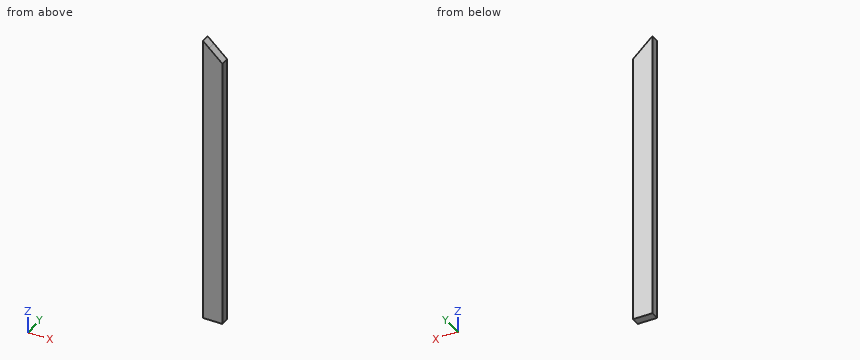
```python
from build123d import *

# Parameters (mm, degrees)
F0_W     = 88.9
F0_H     = 38.1
F1_DEPTH = 1371.6
F3_DEPTH = 38.101


with BuildPart() as f1:
    # F0 (on Top) → F1 (new body)
    with BuildSketch(Plane.XY):
        with Locations((44.45, 19.05)):
            Rectangle(F0_W, F0_H)
    extrude(amount=F1_DEPTH)

    # F2 (on face) → F3 (cut, through all)
    with BuildSketch(Plane.XZ):
        Polygon((28.53436, 1306.33978), (88.9, 1371.6), (0, 1371.6), (0, 1332.734131), align=None)
        Polygon((88.9, 1250.501419), (88.9, 1371.6), (28.53436, 1306.33978), align=None)
    extrude(amount=-F3_DEPTH, mode=Mode.SUBTRACT)


solid = f1.part
```
Geometry: final body of the model. Coordinates: model frame, mm. Give positions to 0.01 mm unless a question says otherwise; leave off trailing zeros. Write each loop counter-clockwise with the first axis right and the second up, starting at its lowest first coordinate (ties: lowest second). Pieces come first, ordered by that corner, then holes.
1. Pin query (flat end, axial travel): P1, Ø4, axis at x = 67.5, y = 21, coming from the +Z side. Return the tip coordinate at first contact, or that it passes through.
2. Section query A-A, the plane y = 15. Return loops of the section in (x, z), then the cut area to 3 significant figures.
3. Line query: probe 1 along Z at (x, y) = (35.5, 19.5); probe 2 along Z at (x, y) = (55, 18). Output: solid intervals per line, ascending.
4. Section query B-B, the plane x = 68. Return loops of the section in (y, z), then the cut area to 3 significant figures.
Computed:
1. P1: stops at z = 1272.15
2. outline: (0, 0) - (88.9, 0) - (88.9, 1250.5) - (0, 1332.73) - close
2. area: 115,000 mm2
3. probe 1: z = 0 to 1299.9
3. probe 2: z = 0 to 1281.86
4. outline: (0, 0) - (38.1, 0) - (38.1, 1269.83) - (0, 1269.83) - close
4. area: 48,400 mm2
